Check sheet for the modelled part. Datum: model origin and axes. Units: mm. A direction names the side the tool comes from. Give positions to 0.01 mm unless a question says otherwise; leave off trailing zeros. Write each loop counter-clockwise with the first axis right and the second up, starting at its lowest first coordinate (ties: lowest second). Pieces come first, ordered by that corner, then holes. Notation, with made-up numbers: (-3.75, -7) -> (44.25, -7) arc R22 ccw to (44.25, 12) -> close; hole circle Ø5 at (-15.5, -3). An arc over 180 degrees is marked (long way). Use a Markdown table: item, result. Add a question column.
1. Cross-section at A-A (z = 113). Enter the section's corners in (x, y), then the cut area to 3 significant figures.
2. Cross-section at C-C (y = 31.5). Enter the section's corners in (x, z).
3. Cross-section at B-B (x = 53.5). Enter the section's corners in (y, z), then the cut area to 3 significant figures.
4. Scan lines: probe 1 along Y at (x, z) = (-7.5, 89); probe 2 along Z at (x, y) = (-25, 113.5). Record each from-to range of solid material in increasing order. Write a range as [from, to].
5. Set-up check for faces 1 (the flat face through (1, 88, -107.5)), 2 (the flat face through (-1, 0, 9)): record each of +Z, -Z, +X, -X, +Y, -Y from which the full face is reachable in a straight line by a thin tool's end or side.
6. Cross-section at D-D (x = -42). Enter the section's corners in (y, z), then the cut area to 3 significant figures.
7. Gauge pin test, flat end, axial feed: P1, Ø12, axis at x = -26.5, z = -7.5, coming from the +Y side. Record the tip position at first contact, or that the pin passes through.
from build123d import *

# Parameters (mm, degrees)
SKETCH1_W          = 125
SKETCH1_H          = 210
BASE_FLANGE1_DEPTH = 0.7
EDGE_FLANGE1_DEPTH = 125
SKETCH9_W          = 12.7
SKETCH9_H          = 23
TAB1_DEPTH         = 0.7
SKETCH12_W         = 12.7
SKETCH12_H         = 23
TAB2_DEPTH         = 0.7


# Sheet-metal steps are written as plain solids
with BuildPart() as part:
    # Sketch1 → Base-Flange1 (new body)
    with BuildSketch(Plane(origin=(0, 0, 0), x_dir=(1, 0, 0), z_dir=(0, 1, 0))):
        Rectangle(SKETCH1_W, SKETCH1_H)
    extrude(amount=-BASE_FLANGE1_DEPTH)

    # Edge-Flange1 section (across the edge) → Edge-Flange1 (add)
    with BuildSketch(Plane(origin=(62.5, 0, -106.8), x_dir=(0, 0, 1), z_dir=(-1, 0, 0))):
        with BuildLine():
            Line((-0.7, 1), (-0.7, 177.1))
            Line((-0.7, 177.1), (0, 177.1))
            Line((0, 177.1), (0, 1))
            ThreePointArc((0, 1), (0.292893219, 0.292893219), (1, 0))
            Line((1, 0), (1.8, 0))
            Line((1.8, 0), (1.8, -0.7))
            Line((1.8, -0.7), (1, -0.7))
            ThreePointArc((1, -0.7), (-0.202081528, -0.202081528), (-0.7, 1))
        make_face()
    extrude(amount=EDGE_FLANGE1_DEPTH)

    # Sketch9 → Tab1 (add)
    with BuildSketch(Plane(origin=(0, 0, 0), x_dir=(1, 0, 0), z_dir=(0, 1, 0))):
        with Locations((-56.15, -116.5)):
            Rectangle(SKETCH9_W, SKETCH9_H)
    extrude(amount=-TAB1_DEPTH)

    # Sketch12 → Tab2 (add)
    with BuildSketch(Plane(origin=(0, 0, 0), x_dir=(1, 0, 0), z_dir=(0, 1, 0))):
        with Locations((56.15, -116.5)):
            Rectangle(SKETCH12_W, SKETCH12_H)
    extrude(amount=-TAB2_DEPTH)


solid = part.part
Worked answers:
| question | item | result |
|---|---|---|
| 1 | outline | (-62.5, -0.7) -> (-49.8, -0.7) -> (-49.8, 0) -> (-62.5, 0) -> close; (49.8, -0.7) -> (62.5, -0.7) -> (62.5, 0) -> (49.8, 0) -> close |
| 1 | area | 17.8 mm² |
| 2 | outline | (-62.5, -107.5) -> (62.5, -107.5) -> (62.5, -106.8) -> (-62.5, -106.8) -> close |
| 3 | outline | (-0.7, -105.8) arc R1.7 ccw to (1, -107.5) -> (177.1, -107.5) -> (177.1, -106.8) -> (1, -106.8) arc R1 cw to (0, -105.8) -> (0, 128) -> (-0.7, 128) -> close |
| 3 | area | 288 mm² |
| 4 | probe 1 | y = [-0.7, 0] |
| 4 | probe 2 | z = [-107.5, -106.8] |
| 5 | face 1 | -Z, +X, -X, +Y, -Y |
| 5 | face 2 | +Z, +X, -X, +Y |
| 6 | outline | (-0.7, -105.8) arc R1.7 ccw to (1, -107.5) -> (177.1, -107.5) -> (177.1, -106.8) -> (1, -106.8) arc R1 cw to (0, -105.8) -> (0, 105) -> (-0.7, 105) -> close |
| 6 | area | 272 mm² |
| 7 | P1 | stops at y = 0 |
